Model file for the job. Use its own axes, mm. A direction names the side the tool comes from. Round coordinates to 2 decimals unless told otherwise and drop trailing zeros. Order: outer loops, then holes, each group sorted by start corner. A loop starts at its lowest first (then second) coordinate and runs counter-clockwise, first axis right, second up. Notation, with made-up numbers: (4, 64.5) - (23, 64.5) arc R11 cw to (23, 69.5) - close; hole circle Ø10 at (54.5, -23). An arc over 180 degrees is marked (long way). Answer as CSV lines item,"result". Start each with the question number.
1. Band-saw the part on D-D on x = 5. State how many separate pieces and enclosed holes the cut face has, then the cut area to 3 significant figures.
2. Pull direction X, two halves, no side cores. Call faces 5 (the face through (5.75, 51.09, 2.64)), 6 (the face through (2, 43, -2)), 7 (the face through (-6.421, 61.535, -3.845)), 8 (the face through (10, 46, 3.2)): released by +X, released by -X, zero draft, split by the parting line, or undercut.
3. Wall check: line 1 along Y through (x, z) = (-2, 8); line 2 along X through (y, z) = (61.55, -3); line 3 along Z through (x, y) = (-5.5, 60.9). Give the ranges that are in metal, low to high. Write a range as [from, to].
4. 3-axis set-ups, long thin cutter, end or side, ignore diameter. For faces 1 (the face through (3.409, 56.605, -6.115)), 2 (the face through (-4, 49, 6)), 3 (the face through (-3.59, 56.6, 6.01)), 4 (the face through (5.317, 58.746, 3.248)): which of +Z, -Z, +X, -X, +Y, -Y reach the whole face in a straight line?
5. Pin check, flat tips, straight feed: pin 1 Ø3 at (x, y) = (5.5, 55.5) entering from +Z; pin 2 Ø12 at (y, z) = (53, -7) entering from -X; pin 3 Ø8 at (y, z) = (55.5, 1) entering from +X. Stop position of each tip, or through.
6. Band-saw the part on B-B on y = 47.5. List the corners of the cut face in (x, z).
7. Band-saw the part on C-C on z = -5. List the corners of the cut face in (x, y), then the cut area to 3 significant figures.
8. Band-saw the part on A-A on x = -1. List the corners of the cut face in (y, z).
```python
from build123d import *

# Parameters (mm, degrees)
SKETCH001_R    = 10.5
SKETCH001_R_2  = 2.55
PAD001_DEPTH   = 21
SKETCH003_R    = 20.618255
POCKET_DEPTH   = 15
SKETCH015_R    = 1.25
HOLE004_DEPTH  = 5
HOLE004_TIPS_R = 1.25
SKETCH039_R    = 1.25
HOLE011_DEPTH  = 10
HOLE011_TIPS_R = 1.25


with BuildPart() as part:
    # Sketch001 → Pad001 (new body)
    with BuildSketch(Plane.XZ):
        Circle(SKETCH001_R)
        Circle(SKETCH001_R_2, mode=Mode.SUBTRACT)
    extrude(amount=PAD001_DEPTH)

    # Sketch003 (on Face3 of Pad001) → Pocket (cut)
    with BuildSketch(Plane(origin=(0, 0, 0), x_dir=(1, 0, 0), z_dir=(0, 1, 0))):
        Circle(SKETCH003_R)
        with BuildLine():
            ThreePointArc((-3.1024143311, 9.8740835179), (-8.9633629292, 5.175), (-10.1024143311, -2.2502721351))
            Line((-10.1024143311, -2.2502721351), (3.1044730766, -9.8752721351))
            ThreePointArc((3.1044730766, -9.8752721351), (8.9648795095, -5.175875598), (10.1044730766, 2.2490835179))
            Line((-3.1024143311, 9.8740835179), (10.1044730766, 2.2490835179))
        make_face(mode=Mode.SUBTRACT)
    extrude(amount=-POCKET_DEPTH, mode=Mode.SUBTRACT)

    # Sketch015 (on Face9 of Pocket) → Hole004 (cut)
    with BuildSketch(Plane(origin=(0, 0, 0), x_dir=(1, 0, 0), z_dir=(0, 1, 0))):
        with Locations((-5.5, 3)):
            Circle(SKETCH015_R)
    extrude(amount=-HOLE004_DEPTH, mode=Mode.SUBTRACT)

    # Hole004 tips → Hole004 tip 1 section 0
    with BuildSketch(Plane(origin=(0, -5, 0), x_dir=(1, 0, 0), z_dir=(0, 1, 0)), mode=Mode.PRIVATE) as hole004_tip_1_s0:
        with Locations((-5.5, 3)):
            Circle(HOLE004_TIPS_R)
    loft([hole004_tip_1_s0.sketch, Vertex(-5.5, -5.7510757738, -3)], mode=Mode.SUBTRACT)

    # Sketch039 (on DatumPlane) → Hole011 (cut)
    with BuildSketch(Plane(origin=(2, 0, 0), x_dir=(0.5, 0, -0.8660254038), z_dir=(-0.8660254038, 0, -0.5))):
        with Locations((-0.991399, 14.019394)):
            Circle(SKETCH039_R)
        with Locations((-0.991399, 4.014446)):
            Circle(SKETCH039_R)
    extrude(amount=-HOLE011_DEPTH, mode=Mode.SUBTRACT)

    # Hole011 tips → Hole011 tip 1 section 0
    with BuildSketch(Plane(origin=(10.6602540378, 0, 5), x_dir=(0.5, 0, -0.8660254038), z_dir=(-0.8660254038, 0, -0.5)), mode=Mode.PRIVATE) as hole011_tip_1_s0:
        with Locations((-0.991399, 14.019394)):
            Circle(HOLE011_TIPS_R)
    loft([hole011_tip_1_s0.sketch, Vertex(10.8150052381, -14.019394, 6.2341146062)], mode=Mode.SUBTRACT)

    # Hole011 tips → Hole011 tip 2 section 0
    with BuildSketch(Plane(origin=(10.6602540378, 0, 5), x_dir=(0.5, 0, -0.8660254038), z_dir=(-0.8660254038, 0, -0.5)), mode=Mode.PRIVATE) as hole011_tip_2_s0:
        with Locations((-0.991399, 4.014446)):
            Circle(HOLE011_TIPS_R)
    loft([hole011_tip_2_s0.sketch, Vertex(10.8150052381, -4.014446, 6.2341146062)], mode=Mode.SUBTRACT)


with BuildPart() as part_1:
    # Body001 placement: moved
    add(part.part.moved(Location((0, 64, 0))))


solid = part_1.part
```
Reply:
1,separate pieces,"1"
1,enclosed holes,"2"
1,area,"313 mm2"
2,face 5,"undercut"
2,face 6,"zero draft"
2,face 7,"undercut"
2,face 8,"split by the parting line"
3,line 1,"y = [43, 49]"
3,line 2,"x = [-9.91, -6.75], [-4.25, 8.8]"
3,line 3,"z = [-8.77, -4.25], [-1.75, 4.91]"
4,face 1,"-Z, +X, +Y"
4,face 2,"+Y"
4,face 3,"+Z, -X, +Y"
4,face 4,"none"
5,pin 1,"stops at z = 9.55"
5,pin 2,"stops at x = -10.3"
5,pin 3,"stops at x = 10.35"
6,outline,"circle Ø21 at (0, 0); hole circle Ø5.1 at (0, 0)"
7,outline,"(-9.23, 43) - (9.23, 43) - (9.23, 49) - (5.34, 49) - (5.34, 64) - (-9.06, 64) - (-9.06, 49) - (-9.23, 49) - close"
7,area,"327 mm2"
8,outline,"(43, -10.45) - (49, -10.45) - (49, -8.66) - (64, -8.66) - (64, -2.35) - (43, -2.35) - close; (43, 2.35) - (64, 2.35) - (64, 7.51) - (49, 7.51) - (49, 10.45) - (43, 10.45) - close"
